For this review, use the dimensioned drawing (mm, ordinates from the lowest corner) and the shaded views. A direction names the side the tool comes from. Give positions to 0.01 mm unless a question says otherwise; leave off trailing zeros. Order: outer loops, then holes, each group sorted by start corner. A loop starts at its lowest first (then second) coordinate and runs counter-clockwise, first axis right, second up. Notation, with made-up numbers: (56.25, -2.75) -> (78.25, -2.75) arc R10 ccw to (78.25, 11.25) -> close; hole circle Ø7 at (-31, 21.5). An arc over 180 degrees is marked (long way). Answer as a JSON object with one key per item and string values. Group by question number.
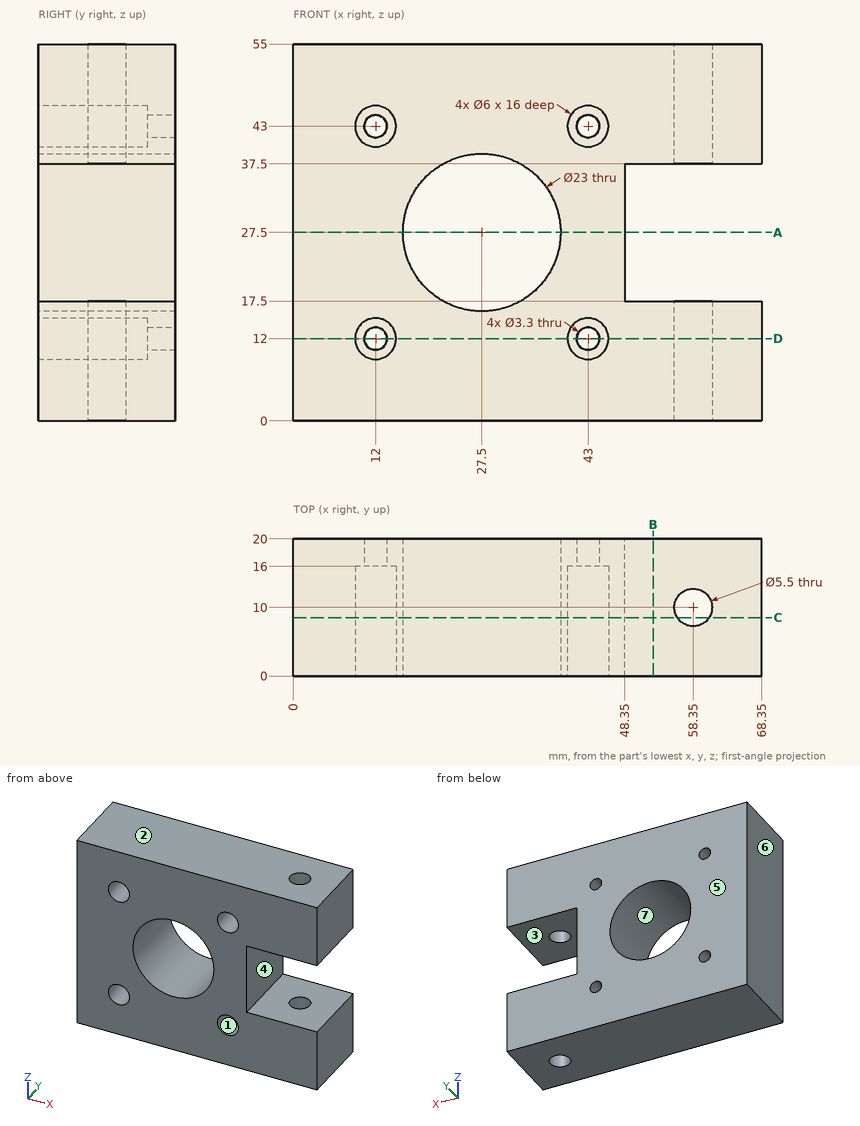
1. Take a section at D-D on z = 12. Give the boundary of the cut face in (x, y), plus the area to 3 significant figures.
2. Take a section at B-B on x = 52.5. Give the boundary of the cut face in (y, z), plus the area to 3 significant figures.
3. Machinability: for the marked faces 1, 2 and 3, which of the approach directions +Z, -Z, +X, -X, +Y, -Y give a long, thin tool a straight path to every point of the face, cutting with its end or side? Answer none if there is none.
4. Take a section at A-A on z = 27.5. Give the boundary of the cut face in (x, y), plus the area to 3 significant figures.
5. Draft analysis for pull direction X (two halves, no side actions). For the marked faces 4, 5, 6 and 7, state which applies: pulls with the +X half, pulls with the -X half, needs draft (parallel to the pull), parting line crosses it, or undercut.
6. For pin 1 (5 mm diameter, centred on y = 14, z = 19, fed in from -X); pin 2 (1.8 mm diameter, centred on x = 42, z = 10.5, fed in from -Y); pin 3 (2.5 mm diameter, centred on x = 12, z = 43, fed in from +Y); pin 4 (1.5 mm diameter, centred on y = 12, z = 30, fed in from +X), all flat-tipped, find the tip position at first contact; note any pin that passes through.
7. Take a section at C-C on y = 8.5. Give the boundary of the cut face in (x, z).
8. For probe 1 along X at (y, z) = (18.5, 43); probe 2 along X at (y, z) = (9.75, 43); probe 3 along Z at (x, y) = (12, 17.5), list the stretches that pass through material, from the lowest coordinate up. Write a range as [from, to].
Checks:
{
 "1": {"outline": "(0, 0) -> (9, 0) -> (9, 16) -> (10.35, 16) -> (10.35, 20) -> (0, 20) -> close; (13.65, 16) -> (15, 16) -> (15, 0) -> (40, 0) -> (40, 16) -> (41.35, 16) -> (41.35, 20) -> (13.65, 20) -> close; (44.65, 16) -> (46, 16) -> (46, 0) -> (68.35, 0) -> (68.35, 20) -> (44.65, 20) -> close; hole circle Ø5.5 at (58.35, 10)", "area": "1,120 mm2"},
 "2": {"outline": "(0, 0) -> (20, 0) -> (20, 17.5) -> (0, 17.5) -> close; (0, 37.5) -> (20, 37.5) -> (20, 55) -> (0, 55) -> close", "area": "700 mm2"},
 "3": {"face 1": "-Y", "face 2": "+Z, +X, -X, +Y, -Y", "face 3": "+X, +Y, -Y"},
 "4": {"outline": "(0, 0) -> (16, 0) -> (16, 20) -> (0, 20) -> close; (39, 0) -> (48.35, 0) -> (48.35, 20) -> (39, 20) -> close", "area": "507 mm2"},
 "5": {"face 4": "pulls with the +X half", "face 5": "needs draft", "face 6": "pulls with the -X half", "face 7": "undercut"},
 "6": {"pin 1": "stops at x = 0", "pin 2": "stops at y = 16", "pin 3": "passes through", "pin 4": "stops at x = 48.35"},
 "7": {"outline": "(0, 0) -> (56.05, 0) -> (56.05, 17.5) -> (48.35, 17.5) -> (48.35, 37.5) -> (56.05, 37.5) -> (56.05, 55) -> (0, 55) -> close; (60.65, 0) -> (68.35, 0) -> (68.35, 17.5) -> (60.65, 17.5) -> close; (60.65, 37.5) -> (68.35, 37.5) -> (68.35, 55) -> (60.65, 55) -> close; hole circle Ø6 at (12, 12); hole circle Ø6 at (12, 43); hole circle Ø23 at (27.5, 27.5); hole circle Ø6 at (43, 12); hole circle Ø6 at (43, 43)"},
 "8": {"probe 1": "x = [0, 10.35], [13.65, 41.35], [44.65, 68.35]", "probe 2": "x = [0, 9], [15, 40], [46, 55.61], [61.09, 68.35]", "probe 3": "z = [0, 10.35], [13.65, 41.35], [44.65, 55]"}
}
